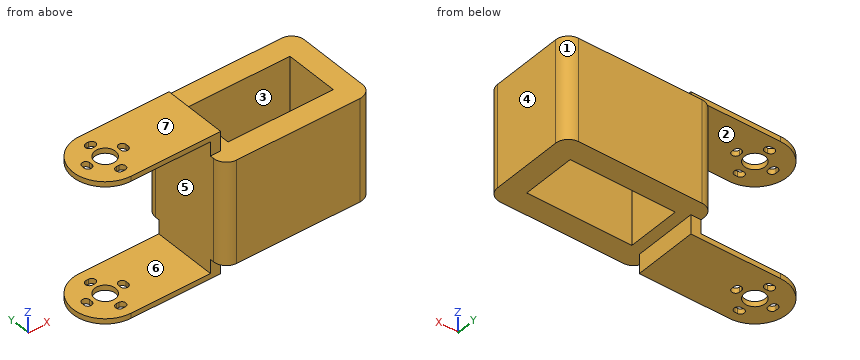
from build123d import *

# Parameters (mm, degrees)
SKETCH1_W           = 58
SKETCH1_H           = 38
SKETCH1_W_2         = 41
SKETCH1_H_2         = 21
BOSS_EXTRUDE1_DEPTH = 40
SKETCH2_W           = 4
SKETCH2_H           = 25
BOSS_EXTRUDE2_DEPTH = 5.55
SKETCH2_2_W         = 4
SKETCH2_2_H         = 25
BOSS_EXTRUDE3_DEPTH = 45.55
SKETCH3_W           = 4
SKETCH3_H           = 25
BOSS_EXTRUDE6_DEPTH = 2
BOSS_EXTRUDE7_START = -53
SKETCH3_8_W         = 4
SKETCH3_8_H         = 25
BOSS_EXTRUDE7_DEPTH = 53
CUT_EXTRUDE1_START  = -51
CUT_EXTRUDE1_DEPTH  = 51
FILLET2_R           = 5
FILLET3_R           = 5
FILLET4_R           = 5
FILLET5_R           = 5


with BuildPart() as part:
    # Sketch1 → Boss-Extrude1 (new body)
    with BuildSketch(Plane.XY):
        with Locations((-0.095837804, -6.136072895)):
            Rectangle(SKETCH1_W, SKETCH1_H)
        with Locations((-0.095837804, -6.136072895)):
            Rectangle(SKETCH1_W_2, SKETCH1_H_2, mode=Mode.SUBTRACT)
    extrude(amount=BOSS_EXTRUDE1_DEPTH)

    # Sketch2 → Boss-Extrude2 (add)
    with BuildSketch(Plane.XY.offset(40)):
        with Locations((-27.095837804, -6.136072895)):
            Rectangle(SKETCH2_W, SKETCH2_H)
    extrude(amount=BOSS_EXTRUDE2_DEPTH)

    # Sketch2_2 → Boss-Extrude3 (add)
    with BuildSketch(Plane.XY.offset(40)):
        with Locations((-27.095837804, -6.136072895)):
            Rectangle(SKETCH2_2_W, SKETCH2_2_H)
    extrude(amount=-BOSS_EXTRUDE3_DEPTH)

    # Sketch3 → Boss-Extrude6 (add)
    # profile 1 of 3: a face of its own
    with BuildSketch(Plane.XY.offset(45.55)):
        with BuildLine():
            Line((-60.095837804, 2.463927105), (-60.095837804, 6.363927105))
            ThreePointArc((-60.095837804, 6.363927105), (-72.595837804, -6.136072895), (-60.095837804, -18.636072895))
            Line((-60.095837804, -18.636072895), (-60.095837804, -15.176248856))
            Line((-60.095837804, -15.176248856), (-60.555926168, -15.176248856))
            ThreePointArc((-60.555926168, -15.176248856), (-62.055926168, -13.676248856), (-60.555926168, -12.176248856))
            Line((-60.555926168, -12.176248856), (-60.095837804, -12.176248856))
            Line((-60.095837804, -12.176248856), (-60.095837804, -10.186072895))
            ThreePointArc((-60.095837804, -10.186072895), (-64.145837804, -6.136072895), (-60.095837804, -2.086072895))
            Line((-60.095837804, -2.086072895), (-60.095837804, -0.536072895))
            Line((-60.095837804, -0.536072895), (-60.595837804, -0.536072895))
            ThreePointArc((-60.595837804, -0.536072895), (-62.095837804, 0.963927105), (-60.595837804, 2.463927105))
            Line((-60.595837804, 2.463927105), (-60.095837804, 2.463927105))
        make_face()
        with BuildLine():
            ThreePointArc((-68.695837804, -5.636072895), (-67.195837804, -4.136072895), (-65.695837804, -5.636072895))
            Line((-65.695837804, -5.636072895), (-65.695837804, -6.636072895))
            ThreePointArc((-65.695837804, -6.636072895), (-67.195837804, -8.136072895), (-68.695837804, -6.636072895))
            Line((-68.695837804, -6.636072895), (-68.695837804, -5.636072895))
        make_face(mode=Mode.SUBTRACT)
    # profile 2 of 3: a face of its own
    with BuildSketch(Plane.XY.offset(45.55)):
        with BuildLine():
            Line((-29.095837804, -18.636072895), (-29.095837804, 6.363927105))
            Line((-29.095837804, 6.363927105), (-60.095837804, 6.363927105))
            Line((-60.095837804, 6.363927105), (-60.095837804, 2.463927105))
            Line((-60.095837804, 2.463927105), (-59.595837804, 2.463927105))
            ThreePointArc((-59.595837804, 2.463927105), (-58.095837804, 0.963927105), (-59.595837804, -0.536072895))
            Line((-59.595837804, -0.536072895), (-60.095837804, -0.536072895))
            Line((-60.095837804, -0.536072895), (-60.095837804, -2.086072895))
            ThreePointArc((-60.095837804, -2.086072895), (-57.23205534, -3.272290432), (-56.045837804, -6.136072895))
            ThreePointArc((-56.045837804, -6.136072895), (-57.23205534, -8.999855359), (-60.095837804, -10.186072895))
            Line((-60.095837804, -10.186072895), (-60.095837804, -12.176248856))
            Line((-60.095837804, -12.176248856), (-59.635749439, -12.176248856))
            ThreePointArc((-59.635749439, -12.176248856), (-58.135749439, -13.676248856), (-59.635749439, -15.176248856))
            Line((-59.635749439, -15.176248856), (-60.095837804, -15.176248856))
            Line((-60.095837804, -15.176248856), (-60.095837804, -18.636072895))
            Line((-60.095837804, -18.636072895), (-29.095837804, -18.636072895))
        make_face()
        with BuildLine():
            ThreePointArc((-54.495837804, -5.636072895), (-52.995837804, -4.136072895), (-51.495837804, -5.636072895))
            Line((-51.495837804, -5.636072895), (-51.495837804, -6.636072895))
            ThreePointArc((-51.495837804, -6.636072895), (-52.995837804, -8.136072895), (-54.495837804, -6.636072895))
            Line((-54.495837804, -6.636072895), (-54.495837804, -5.636072895))
        make_face(mode=Mode.SUBTRACT)
    # profile 3 of 3: a face of its own
    with BuildSketch(Plane.XY.offset(45.55)):
        with Locations((-27.095837804, -6.136072895)):
            Rectangle(SKETCH3_W, SKETCH3_H)
    extrude(amount=BOSS_EXTRUDE6_DEPTH)

    # Sketch3_8 → Boss-Extrude7 (add)
    # profile 1 of 3: a face of its own
    with BuildSketch(Plane.XY.offset(45.55).offset(BOSS_EXTRUDE7_START)):
        with BuildLine():
            Line((-60.095837804, 2.463927105), (-60.095837804, 6.363927105))
            ThreePointArc((-60.095837804, 6.363927105), (-72.595837804, -6.136072895), (-60.095837804, -18.636072895))
            Line((-60.095837804, -18.636072895), (-60.095837804, -15.176248856))
            Line((-60.095837804, -15.176248856), (-60.555926168, -15.176248856))
            ThreePointArc((-60.555926168, -15.176248856), (-62.055926168, -13.676248856), (-60.555926168, -12.176248856))
            Line((-60.555926168, -12.176248856), (-60.095837804, -12.176248856))
            Line((-60.095837804, -12.176248856), (-60.095837804, -10.186072895))
            ThreePointArc((-60.095837804, -10.186072895), (-64.145837804, -6.136072895), (-60.095837804, -2.086072895))
            Line((-60.095837804, -2.086072895), (-60.095837804, -0.536072895))
            Line((-60.095837804, -0.536072895), (-60.595837804, -0.536072895))
            ThreePointArc((-60.595837804, -0.536072895), (-62.095837804, 0.963927105), (-60.595837804, 2.463927105))
            Line((-60.595837804, 2.463927105), (-60.095837804, 2.463927105))
        make_face()
        with BuildLine():
            ThreePointArc((-68.695837804, -5.636072895), (-67.195837804, -4.136072895), (-65.695837804, -5.636072895))
            Line((-65.695837804, -5.636072895), (-65.695837804, -6.636072895))
            ThreePointArc((-65.695837804, -6.636072895), (-67.195837804, -8.136072895), (-68.695837804, -6.636072895))
            Line((-68.695837804, -6.636072895), (-68.695837804, -5.636072895))
        make_face(mode=Mode.SUBTRACT)
    # profile 2 of 3: a face of its own
    with BuildSketch(Plane.XY.offset(45.55).offset(BOSS_EXTRUDE7_START)):
        with BuildLine():
            Line((-29.095837804, -18.636072895), (-29.095837804, 6.363927105))
            Line((-29.095837804, 6.363927105), (-60.095837804, 6.363927105))
            Line((-60.095837804, 6.363927105), (-60.095837804, 2.463927105))
            Line((-60.095837804, 2.463927105), (-59.595837804, 2.463927105))
            ThreePointArc((-59.595837804, 2.463927105), (-58.095837804, 0.963927105), (-59.595837804, -0.536072895))
            Line((-59.595837804, -0.536072895), (-60.095837804, -0.536072895))
            Line((-60.095837804, -0.536072895), (-60.095837804, -2.086072895))
            ThreePointArc((-60.095837804, -2.086072895), (-57.23205534, -3.272290432), (-56.045837804, -6.136072895))
            ThreePointArc((-56.045837804, -6.136072895), (-57.23205534, -8.999855359), (-60.095837804, -10.186072895))
            Line((-60.095837804, -10.186072895), (-60.095837804, -12.176248856))
            Line((-60.095837804, -12.176248856), (-59.635749439, -12.176248856))
            ThreePointArc((-59.635749439, -12.176248856), (-58.135749439, -13.676248856), (-59.635749439, -15.176248856))
            Line((-59.635749439, -15.176248856), (-60.095837804, -15.176248856))
            Line((-60.095837804, -15.176248856), (-60.095837804, -18.636072895))
            Line((-60.095837804, -18.636072895), (-29.095837804, -18.636072895))
        make_face()
        with BuildLine():
            ThreePointArc((-54.495837804, -5.636072895), (-52.995837804, -4.136072895), (-51.495837804, -5.636072895))
            Line((-51.495837804, -5.636072895), (-51.495837804, -6.636072895))
            ThreePointArc((-51.495837804, -6.636072895), (-52.995837804, -8.136072895), (-54.495837804, -6.636072895))
            Line((-54.495837804, -6.636072895), (-54.495837804, -5.636072895))
        make_face(mode=Mode.SUBTRACT)
    # profile 3 of 3: a face of its own
    with BuildSketch(Plane.XY.offset(45.55).offset(BOSS_EXTRUDE7_START)):
        with Locations((-27.095837804, -6.136072895)):
            Rectangle(SKETCH3_8_W, SKETCH3_8_H)
    extrude(amount=BOSS_EXTRUDE7_DEPTH)

    # Sketch3_11 → Cut-Extrude1 (cut)
    # profile 1 of 2: a face of its own
    with BuildSketch(Plane.XY.offset(45.55).offset(CUT_EXTRUDE1_START)):
        with BuildLine():
            Line((-29.095837804, -18.636072895), (-29.095837804, 6.363927105))
            Line((-29.095837804, 6.363927105), (-60.095837804, 6.363927105))
            Line((-60.095837804, 6.363927105), (-60.095837804, 2.463927105))
            Line((-60.095837804, 2.463927105), (-59.595837804, 2.463927105))
            ThreePointArc((-59.595837804, 2.463927105), (-58.095837804, 0.963927105), (-59.595837804, -0.536072895))
            Line((-59.595837804, -0.536072895), (-60.095837804, -0.536072895))
            Line((-60.095837804, -0.536072895), (-60.095837804, -2.086072895))
            ThreePointArc((-60.095837804, -2.086072895), (-57.23205534, -3.272290432), (-56.045837804, -6.136072895))
            ThreePointArc((-56.045837804, -6.136072895), (-57.23205534, -8.999855359), (-60.095837804, -10.186072895))
            Line((-60.095837804, -10.186072895), (-60.095837804, -12.176248856))
            Line((-60.095837804, -12.176248856), (-59.635749439, -12.176248856))
            ThreePointArc((-59.635749439, -12.176248856), (-58.135749439, -13.676248856), (-59.635749439, -15.176248856))
            Line((-59.635749439, -15.176248856), (-60.095837804, -15.176248856))
            Line((-60.095837804, -15.176248856), (-60.095837804, -18.636072895))
            Line((-60.095837804, -18.636072895), (-29.095837804, -18.636072895))
        make_face()
        with BuildLine():
            ThreePointArc((-54.495837804, -5.636072895), (-52.995837804, -4.136072895), (-51.495837804, -5.636072895))
            Line((-51.495837804, -5.636072895), (-51.495837804, -6.636072895))
            ThreePointArc((-51.495837804, -6.636072895), (-52.995837804, -8.136072895), (-54.495837804, -6.636072895))
            Line((-54.495837804, -6.636072895), (-54.495837804, -5.636072895))
        make_face(mode=Mode.SUBTRACT)
    # profile 2 of 2: a face of its own
    with BuildSketch(Plane.XY.offset(45.55).offset(CUT_EXTRUDE1_START)):
        with BuildLine():
            Line((-60.095837804, 2.463927105), (-60.095837804, 6.363927105))
            ThreePointArc((-60.095837804, 6.363927105), (-72.595837804, -6.136072895), (-60.095837804, -18.636072895))
            Line((-60.095837804, -18.636072895), (-60.095837804, -15.176248856))
            Line((-60.095837804, -15.176248856), (-60.555926168, -15.176248856))
            ThreePointArc((-60.555926168, -15.176248856), (-62.055926168, -13.676248856), (-60.555926168, -12.176248856))
            Line((-60.555926168, -12.176248856), (-60.095837804, -12.176248856))
            Line((-60.095837804, -12.176248856), (-60.095837804, -10.186072895))
            ThreePointArc((-60.095837804, -10.186072895), (-64.145837804, -6.136072895), (-60.095837804, -2.086072895))
            Line((-60.095837804, -2.086072895), (-60.095837804, -0.536072895))
            Line((-60.095837804, -0.536072895), (-60.595837804, -0.536072895))
            ThreePointArc((-60.595837804, -0.536072895), (-62.095837804, 0.963927105), (-60.595837804, 2.463927105))
            Line((-60.595837804, 2.463927105), (-60.095837804, 2.463927105))
        make_face()
        with BuildLine():
            ThreePointArc((-68.695837804, -5.636072895), (-67.195837804, -4.136072895), (-65.695837804, -5.636072895))
            Line((-65.695837804, -5.636072895), (-65.695837804, -6.636072895))
            ThreePointArc((-65.695837804, -6.636072895), (-67.195837804, -8.136072895), (-68.695837804, -6.636072895))
            Line((-68.695837804, -6.636072895), (-68.695837804, -5.636072895))
        make_face(mode=Mode.SUBTRACT)
    extrude(amount=CUT_EXTRUDE1_DEPTH, mode=Mode.SUBTRACT)

    # Fillet2
    fillet2_edges = [part.edges().sort_by_distance(p)[0] for p in [
        (28.904162196, 12.863927105, 20),
    ]]
    fillet(fillet2_edges, radius=FILLET2_R)

    # Fillet3
    fillet3_edges = [part.edges().sort_by_distance(p)[0] for p in [
        (28.904162196, -25.136072895, 20),
    ]]
    fillet(fillet3_edges, radius=FILLET3_R)

    # Fillet4
    fillet4_edges = [part.edges().sort_by_distance(p)[0] for p in [
        (-29.095837804, 12.863927105, 20),
    ]]
    fillet(fillet4_edges, radius=FILLET4_R)

    # Fillet5
    fillet5_edges = [part.edges().sort_by_distance(p)[0] for p in [
        (-29.095837804, -25.136072895, 20),
    ]]
    fillet(fillet5_edges, radius=FILLET5_R)


solid = part.part
Work out the finished part from the listing and answer in its coordinate system (mm). Face numbers are marked on the shaded views. A direction names the side the tool comes from. Coordinates: 2 decimals unless noted, no trailing zeros. Write each loop counter-clockwise with the first axis right and the second up, starting at its lowest first coordinate (ties: lowest second). Pieces come first, ordered by that corner, then holes. Notation, with made-up numbers: M -11.75,26.25 L 27.25,26.25 A32 cw 27.25,57.25 Z; hole C -23,7.5 d11. An arc over 180 degrees is marked long. Answer as CSV lines item,"result". Start each with the question number.
Item 1: A tool of negligible diameter and unlimited length cuts with its end or side. For the marked faces 1, 2 and 3, from which of +Z, -Z, +X, -X, +Y, -Y can it reach the whole face along a straight path? Write none if from no direction.
Item 2: Section B-B on z = 28 is taken. Write down the section's boundary in (x, y), and give its area (3 significant figures).
Item 3: Section C-C on y = 1 is taken. Write down the section's boundary in (x, z).
Item 4: Section D-D on z = -4 is taken. Write down the section's boundary in (x, y), and give its area (3 significant figures).
Item 5: Consider L1, parallel to X at y = -11.5, z = 19.5; L2, parallel to Y at x = -17.5, z = 21.5; L3, parallel to Z at x = -36, y = -14.5. Determine where each line is inside the solid, lowest interval first.
Item 6: Flat-ended cylindrical pins translate along their axes: P1, Ø12, axis at y = -9, z = 37, coming from the -X side; P2, Ø1, axis at x = -10, y = -15, coming from the -Z side; P3, Ø0.8, axis at y = -6.5, z = -6.5, coming from the +X side; P4, Ø0.7, axis at x = -60.5, z = -6, coming from the +Y side. Find the tip coordinate at first contact, or state that the pin passes through.
Item 7: Section A-A on x = 9.5 is taken. Write down the section's boundary in (y, z), and give its area (3 significant figures).
Item 8: Determine the mould class of the marked faces 4, 5, 6 and 7 for opening direction Z: released by +Z, released by -Z, zero draft, split by the parting line, or undercut.
Checks:
1,face 1,"+Z, -Z, +X, +Y"
1,face 2,"-X, +Y, -Y"
1,face 3,"+Z, -Z"
2,outline,"M -29.1,-20.14 A5 ccw -24.1,-25.14 L 23.9,-25.14 A5 ccw 28.9,-20.14 L 28.9,7.86 A5 ccw 23.9,12.86 L -24.1,12.86 A5 ccw -29.1,7.86 Z; hole M -20.6,-16.64 L 20.4,-16.64 L 20.4,4.36 L -20.6,4.36 Z"
2,area,"1,320 mm²"
3,outline,"M -70.36,-7.45 L -62.1,-7.45 L -62.1,-5.45 L -70.36,-5.45 Z; M -70.36,45.55 L -62.1,45.55 L -62.1,47.55 L -70.36,47.55 Z; M -58.1,-7.45 L -25.1,-7.45 L -25.1,0 L -20.6,0 L -20.6,40 L -25.1,40 L -25.1,47.55 L -58.1,47.55 L -58.1,45.55 L -29.1,45.55 L -29.1,-5.45 L -58.1,-5.45 Z; M 20.4,0 L 28.9,0 L 28.9,40 L 20.4,40 Z"
4,outline,"M -29.1,-18.64 L -25.1,-18.64 L -25.1,6.36 L -29.1,6.36 Z"
4,area,"100 mm²"
5,L1,"x = -29.1 to -20.6, 20.4 to 28.9"
5,L2,"y = -25.14 to -16.64, 4.36 to 12.86"
5,L3,"z = -7.45 to -5.45, 45.55 to 47.55"
6,P1,"stops at x = -29.1"
6,P2,"passes through"
6,P3,"stops at x = -25.1"
6,P4,"stops at y = 6.36"
7,outline,"M -25.14,0 L -16.64,0 L -16.64,40 L -25.14,40 Z; M 4.36,0 L 12.86,0 L 12.86,40 L 4.36,40 Z"
7,area,"680 mm²"
8,face 4,"zero draft"
8,face 5,"undercut"
8,face 6,"undercut"
8,face 7,"released by +Z"
